from build123d import *

# Parameters (mm, degrees)
F0_R     = 1.6
F0_W     = 20
F0_H     = 8.2
F0_W_2   = 2.2
F0_H_2   = 3.5
F0_W_3   = 3.5
F0_H_3   = 2.1957031846
F1_DEPTH = 2
F0_W_4   = 1.2657215719
F0_H_4   = 1.6254235071
F0_W_5   = 2.1951658177
F0_H_5   = 0.3664782417
F2_DEPTH = 13.9
F3_DEPTH = 8.6
F4_DEPTH = 22.5
F5_R     = 3
F6_DEPTH = 10.2
F7_SIZE2 = 2.0606080646
F7_SIZE  = 0.75
F8_DEPTH = 3.5


with BuildPart() as f1:
    # F0 (on Top) → F1 (new body)
    with BuildSketch(Plane.XY):
        with BuildLine():
            ThreePointArc((35, 30), (33.5355339059, 33.5355339059), (30, 35))
            Line((30, 35), (-30, 35))
            ThreePointArc((-30, 35), (-33.5355339059, 33.5355339059), (-35, 30))
            Line((-35, 30), (-35, -35))
            Line((-35, -35), (35, -35))
            Line((35, -35), (35, 30))
        make_face()
        with Locations((11, -31)):
            Circle(F0_R, mode=Mode.SUBTRACT)
        with Locations((24.4, -29.95)):
            Rectangle(F0_W, F0_H, mode=Mode.SUBTRACT)
        Polygon((-26.2, 20.8), (-26.2, 26.5), (16.4288448244, 26.5), (16.4288448244, 26.5042968154), (19.9288448244, 26.5042968154), (19.9288448244, 26.5), (20, 26.5), (33.1, 13.5), (33.1, -8), (19.3, -8), (5.8042784281, -31.5925206738), (5.8042784281, -31.5945764929), (5.8031024299, -31.5945764929), (5.8, -31.6), (-31.5, -31.6), (-33.1, -29.7), (-33.1, 19.6), (-28.7, 19.6), align=None, mode=Mode.SUBTRACT)
        with Locations((-30, 24)):
            Circle(F0_R, mode=Mode.SUBTRACT)
        with Locations((30, 24)):
            Circle(F0_R, mode=Mode.SUBTRACT)
        Polygon((16.4288448244, 26.5), (-26.2, 26.5), (-26.2, 20.8), (-28.7, 19.6), (-33.1, 19.6), (-33.1, -29.7), (-31.5, -31.6), (5.8, -31.6), (5.8031024299, -31.5945764929), (3.6042784281, -31.5945764929), (3.6042784281, -29.72), (-27.9348341823, -29.72), (-27.9348341823, -31.5535217583), (-31.4348341823, -31.5535217583), (-31.4348341823, -29.3535217583), (-30.13, -29.3535217583), (-30.13, 5.28), (4.87, 5.28), (4.87, -28.0945764929), (5.8042784281, -28.0945764929), (5.8042784281, -31.5925206738), (19.3, -8), (33.1, -8), (33.1, 13.5), (20, 26.5), (19.9288448244, 26.5), (19.9288448244, 24.3042968154), (16.4288448244, 24.3042968154), align=None)
        with Locations((-31.891271472, 6.2)):
            Rectangle(F0_W_2, F0_H_2, mode=Mode.SUBTRACT)
        with Locations((31.9520607591, 11.7002176121)):
            Rectangle(F0_W_2, F0_H_2, mode=Mode.SUBTRACT)
        Polygon((3.6042784281, -28.0945764929), (4.87, -28.0945764929), (4.87, 5.28), (-30.13, 5.28), (-30.13, -29.3535217583), (-27.9348341823, -29.3535217583), (-27.9348341823, -29.72), (3.6042784281, -29.72), align=None)
        with Locations((24.4, -29.95)):
            Rectangle(F0_W, F0_H)
        with Locations((31.9520607591, 11.7002176121)):
            Rectangle(F0_W_2, F0_H_2)
        with Locations((18.1788448244, 25.4021484077)):
            Rectangle(F0_W_3, F0_H_3)
        Polygon((5.8031024299, -31.5945764929), (5.8042784281, -31.5925206738), (5.8042784281, -28.0945764929), (4.87, -28.0945764929), (4.87, -29.72), (3.6042784281, -29.72), (3.6042784281, -31.5945764929), align=None)
        Polygon((-27.9348341823, -31.5535217583), (-27.9348341823, -29.72), (-30.13, -29.72), (-30.13, -29.3535217583), (-31.4348341823, -29.3535217583), (-31.4348341823, -31.5535217583), align=None)
        with Locations((-31.891271472, 6.2)):
            Rectangle(F0_W_2, F0_H_2)
    extrude(amount=-F1_DEPTH)

    # F0 (on Top) → F2 (join)
    with BuildSketch(Plane.XY):
        Polygon((16.4288448244, 26.5), (-26.2, 26.5), (-26.2, 20.8), (-28.7, 19.6), (-33.1, 19.6), (-33.1, -29.7), (-31.5, -31.6), (5.8, -31.6), (5.8031024299, -31.5945764929), (3.6042784281, -31.5945764929), (3.6042784281, -29.72), (-27.9348341823, -29.72), (-27.9348341823, -31.5535217583), (-31.4348341823, -31.5535217583), (-31.4348341823, -29.3535217583), (-30.13, -29.3535217583), (-30.13, 5.28), (4.87, 5.28), (4.87, -28.0945764929), (5.8042784281, -28.0945764929), (5.8042784281, -31.5925206738), (19.3, -8), (33.1, -8), (33.1, 13.5), (20, 26.5), (19.9288448244, 26.5), (19.9288448244, 24.3042968154), (16.4288448244, 24.3042968154), align=None)
        with Locations((-31.891271472, 6.2)):
            Rectangle(F0_W_2, F0_H_2, mode=Mode.SUBTRACT)
        with Locations((31.9520607591, 11.7002176121)):
            Rectangle(F0_W_2, F0_H_2, mode=Mode.SUBTRACT)
        Polygon((3.6042784281, -28.0945764929), (4.87, -28.0945764929), (4.87, 5.28), (-30.13, 5.28), (-30.13, -29.3535217583), (-27.9348341823, -29.3535217583), (-27.9348341823, -29.72), (3.6042784281, -29.72), align=None)
        Polygon((5.8031024299, -31.5945764929), (5.8042784281, -31.5925206738), (5.8042784281, -28.0945764929), (4.87, -28.0945764929), (4.87, -29.72), (3.6042784281, -29.72), (3.6042784281, -31.5945764929), align=None)
        with Locations((-31.891271472, 6.2)):
            Rectangle(F0_W_2, F0_H_2)
        with Locations((18.1788448244, 25.4021484077)):
            Rectangle(F0_W_3, F0_H_3)
        with Locations((31.9520607591, 11.7002176121)):
            Rectangle(F0_W_2, F0_H_2)
        with Locations((4.2371392141, -28.9072882465)):
            Rectangle(F0_W_4, F0_H_4)
        Polygon((-27.9348341823, -31.5535217583), (-27.9348341823, -29.72), (-30.13, -29.72), (-30.13, -29.3535217583), (-31.4348341823, -29.3535217583), (-31.4348341823, -31.5535217583), align=None)
        with Locations((-29.0324170911, -29.5367608792)):
            Rectangle(F0_W_5, F0_H_5)
    extrude(amount=-F2_DEPTH)

    # F0 (on Top) → F3 (join)
    with BuildSketch(Plane.XY):
        with Locations((24.4, -29.95)):
            Rectangle(F0_W, F0_H)
    extrude(amount=-F3_DEPTH)

    # F0 (on Top) → F4 (join)
    with BuildSketch(Plane.XY):
        Polygon((3.6042784281, -28.0945764929), (4.87, -28.0945764929), (4.87, 5.28), (-30.13, 5.28), (-30.13, -29.3535217583), (-27.9348341823, -29.3535217583), (-27.9348341823, -29.72), (3.6042784281, -29.72), align=None)
        with Locations((4.2371392141, -28.9072882465)):
            Rectangle(F0_W_4, F0_H_4)
        with Locations((-29.0324170911, -29.5367608792)):
            Rectangle(F0_W_5, F0_H_5)
    extrude(amount=-F4_DEPTH)

    # F5 (on face) → F6 (join)
    with BuildSketch(Plane(origin=(0, 26.5, 0), x_dir=(-1, 0, 0), z_dir=(0, 1, 0))):
        with Locations((-15.7, -6.8)):
            Circle(F5_R)
    extrude(amount=F6_DEPTH)

    # F7
    f7_edges = [f1.edges().sort_by_distance(p)[0] for p in [
        (18.7, 36.7, -6.8),
    ]]
    f7_side = f1.faces().sort_by_distance((15.7, 36.7, -6.8))[0]
    chamfer(f7_edges, length=F7_SIZE, length2=F7_SIZE2, reference=f7_side)

    # F0 (on Top) → F8 (join)
    with BuildSketch(Plane.XY):
        Polygon((-27.9348341823, -31.5535217583), (-27.9348341823, -29.72), (-30.13, -29.72), (-30.13, -29.3535217583), (-31.4348341823, -29.3535217583), (-31.4348341823, -31.5535217583), align=None)
        Polygon((5.8031024299, -31.5945764929), (5.8042784281, -31.5925206738), (5.8042784281, -28.0945764929), (4.87, -28.0945764929), (4.87, -29.72), (3.6042784281, -29.72), (3.6042784281, -31.5945764929), align=None)
        with Locations((4.2371392141, -28.9072882465)):
            Rectangle(F0_W_4, F0_H_4)
        with Locations((-29.0324170911, -29.5367608792)):
            Rectangle(F0_W_5, F0_H_5)
        with Locations((-31.891271472, 6.2)):
            Rectangle(F0_W_2, F0_H_2)
        with Locations((18.1788448244, 25.4021484077)):
            Rectangle(F0_W_3, F0_H_3)
        with Locations((31.9520607591, 11.7002176121)):
            Rectangle(F0_W_2, F0_H_2)
    extrude(amount=F8_DEPTH)


solid = f1.part
Read the model definition and answer for the solid it produces. Units are mm, in the model's axes. A direction names the side the tool comes from. Give positions to 0.01 mm unless a question says otherwise; leave off trailing zeros. Write each loop counter-clockwise with the first axis right and the second up, starting at its lowest first coordinate (ties: lowest second). Pieces come first, ordered by that corner, then holes. Notation, with made-up numbers: (-33.5, -19) - (9.5, -19) arc R18 cw to (9.5, 13) - close; hole circle Ø10 at (-35, 55). An arc over 180 degrees is marked (long way). Answer in a Markdown table with one row per item. Add a question column.
Item 1: Flat-ended cylindrical pins translate along their axes: P1, Ø2, axis at x = 27.5, z = -6, coming from the +Y side; P2, Ø1, axis at x = 18.5, z = -12.5, coming from the -Y side; P3, Ø8, axis at x = -23, y = -22, coming from the +Z side; P4, Ø3, axis at x = 11, y = -31, coming from the -Z side. Find the tip coordinate at first contact, or state that the pin passes through.
Item 2: Determine the mould class of faces 1 (the face through (26, -8, -8)), 2 (the face through (32, 9.95, 2)), 3 (the face through (33.1, 3, -8)) for opening direction Y: pulls with the +Y half, pulls with the -Y half, needs draft (parallel to the pull), parting line crosses it, or undercut.
Item 3: A tool of negligible diameter and unlimited length cuts with its end or side. For faces 4 (the face through (-30.13, -12, -18)), 5 (the face through (30.852, 12, 2)), 6 (the face through (-26.2, 24, -8)), from which of +Z, -Z, +X, -X, +Y, -Y can it reach the whole face along a straight path? Write none if from no direction.
Item 4: Section D-D, the plane z = -15.75 is taken. Write down the section's boundary in (x, y).
Item 5: Section C-C, the plane x = 11 is taken. Write down the section's boundary in (y, z), and give its area (3 significant figures).
Item 6: Section A-A, the plane x = -9 is taken. Write down the section's boundary in (y, z), and give its area (3 significant figures).
Item 7: Find the intervals of material crossed by L1, parallel to Y at x = 11, z = -0.4; L2, parallel to Y at x = -30, z = -1.1; L3, parallel to Z at x = -13.5, y = 1.5, in increasing order.
Item 8: Section B-B, the plane y = -23 is taken. Write down the section's boundary in (x, z).
Recorded:
| question | item | result |
|---|---|---|
| 1 | P1 | stops at y = 20.05 |
| 1 | P2 | stops at y = -10.27 |
| 1 | P3 | stops at z = 0 |
| 1 | P4 | passes through |
| 2 | face 1 | undercut |
| 2 | face 2 | pulls with the -Y half |
| 2 | face 3 | needs draft |
| 3 | face 4 | -Z, -X, +Y, -Y |
| 3 | face 5 | +Z, -X, +Y, -Y |
| 3 | face 6 | -Z, -X, +Y |
| 4 | outline | (-30.13, -29.72) - (4.87, -29.72) - (4.87, 5.28) - (-30.13, 5.28) - close |
| 5 | outline | (-35, -2) - (-32.6, -2) - (-32.6, 0) - (-35, 0) - close; (-29.4, -2) - (-22.51, -2) - (-22.51, -13.9) - (26.5, -13.9) - (26.5, -2) - (35, -2) - (35, 0) - (-29.4, 0) - close |
| 5 | area | 717 mm2 |
| 6 | outline | (-35, -2) - (-31.6, -2) - (-31.6, -13.9) - (-29.72, -13.9) - (-29.72, -22.5) - (5.28, -22.5) - (5.28, -13.9) - (26.5, -13.9) - (26.5, -2) - (35, -2) - (35, 0) - (-35, 0) - close |
| 6 | area | 1,130 mm2 |
| 7 | L1 | y = -35 to -32.6, -29.4 to 35 |
| 7 | L2 | y = -35 to 22.4, 25.6 to 35 |
| 7 | L3 | z = -22.5 to 0 |
| 8 | outline | (-35, -2) - (-33.1, -2) - (-33.1, -13.9) - (-30.13, -13.9) - (-30.13, -22.5) - (4.87, -22.5) - (4.87, -13.9) - (10.72, -13.9) - (10.72, -2) - (35, -2) - (35, 0) - (-35, 0) - close |
